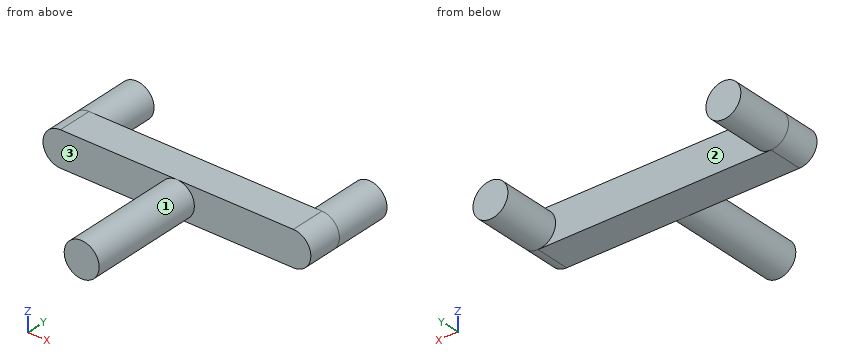
from build123d import *

# Parameters (mm, degrees)
F1_DEPTH = 30
F3_DEPTH = 100
F5_DEPTH = 50


with BuildPart() as f1:
    # F0 (on Front) → F1 (new body)
    with BuildSketch(Plane.XZ):
        with BuildLine():
            Line((100, 15), (-100, 15))
            ThreePointArc((-100, 15), (-115, 0), (-100, -15))
            Line((-100, -15), (100, -15))
            ThreePointArc((100, -15), (115, 0), (100, 15))
        make_face()
    extrude(amount=F1_DEPTH)

    # F2 (on face) → F3 (join)
    with BuildSketch(Plane.XZ.offset(30)):
        with BuildLine():
            ThreePointArc((3.16e-08, -15), (10.606601729, -10.6066017066), (15, 0))
            ThreePointArc((15, 0), (10.6066017178, 10.6066017178), (0, 15))
            ThreePointArc((0, 15), (-15, -1.58e-08), (3.16e-08, -15))
        make_face()
    extrude(amount=F3_DEPTH)

    # F4 (on face) → F5 (join)
    with BuildSketch(Plane(origin=(0, 0, 0), x_dir=(-1, 0, 0), z_dir=(0, 1, 0))):
        with BuildLine():
            ThreePointArc((-100, -15), (-89.3933982822, -10.6066017178), (-85, 0))
            ThreePointArc((-85, 0), (-89.3933982822, 10.6066017178), (-100, 15))
            ThreePointArc((-100, 15), (-115, 0), (-100, -15))
        make_face()
        with BuildLine():
            ThreePointArc((100, 15), (89.3933982822, 10.6066017178), (85, 0))
            ThreePointArc((85, 0), (89.3933982822, -10.6066017178), (100, -15))
            ThreePointArc((100, -15), (110.6066017178, -10.6066017178), (115, 0))
            ThreePointArc((115, 0), (110.6066017178, 10.6066017178), (100, 15))
        make_face()
    extrude(amount=F5_DEPTH)


solid = f1.part
Could you check a few things on this model? Use its own coordinates, in mm. Face numbers are marked on the shaded views. Give positions to 0.01 mm unless a question says otherwise; leave off trailing zeros. Write each loop counter-clockwise with the first axis right and the second up, starting at its lowest first coordinate (ties: lowest second). Pieces come first, ordered by that corner, then holes. Notation, with made-up numbers: (-22, -26) -> (0, -26) arc R17 cw to (0, 2) -> close; hole circle Ø10 at (20, 59). An arc over 180 degrees is marked (long way). Write each question's results on one line, items separated by ' | '. Start each with the question number.
Q1. Suppose I cut it at A-A, the plane y = 37. List the corners of the cut face in (x, z) for me, and give its area (3 significant figures).
Q2. I need wall thicknesses on probe 1 along Y at (x, z) = (22.5, 0); probe 2 along Y at (x, z) = (2.5, 5); probe 3 along Z at (x, y) = (-0.5, -106). Which ranges of each line are inside material? Lowest first, please.
Q3. Suppose I cut it at C-C, the plane x = 51. List the corners of the cut face in (y, z) for me.
Q4. Suppose I cut it at B-B, the plane z = -3. List the corners of the cut face in (x, y) for me, and give its area (3 significant figures).
Q5. Suppose I cut it at D-D, the plane y = -45.5. List the corners of the cut face in (x, z) for me.
Q6. We'd pull the mould along X, two halves only. Please class the marked faces 1, 2 and 3: +X half, -X half, draft (parallel to the pull), parting line (faces both ways), or undercut.
Q7. I'm going to push flat-ended pins straight in: pin 1 Ø1 at (x, z) = (-61, -1.5) entering from -Y; pin 2 Ø4 at (y, z) = (-33.5, -8.5) entering from +X; pin 3 Ø6 at (x, z) = (44, 0.5) entering from +Y. Where does each tip first touch, or does it pass through?
Outcome:
1) outline: circle Ø30 at (-100, 0); circle Ø30 at (100, 0) | area: 1,410 mm2
2) probe 1: -30 to 0 | probe 2: -130 to 0 | probe 3: -14.99 to 14.99
3) outline: (-30, -15) -> (0, -15) -> (0, 15) -> (-30, 15) -> close
4) outline: (-114.7, -30) -> (-14.7, -30) -> (-14.7, -130) -> (14.7, -130) -> (14.7, -30) -> (114.7, -30) -> (114.7, 50) -> (85.3, 50) -> (85.3, 0) -> (-85.3, 0) -> (-85.3, 50) -> (-114.7, 50) -> close | area: 12,800 mm2
5) outline: circle Ø30 at (0, 0)
6) face 1: parting line | face 2: undercut | face 3: draft
7) pin 1: y = -30 | pin 2: x = 13.52 | pin 3: y = 0
